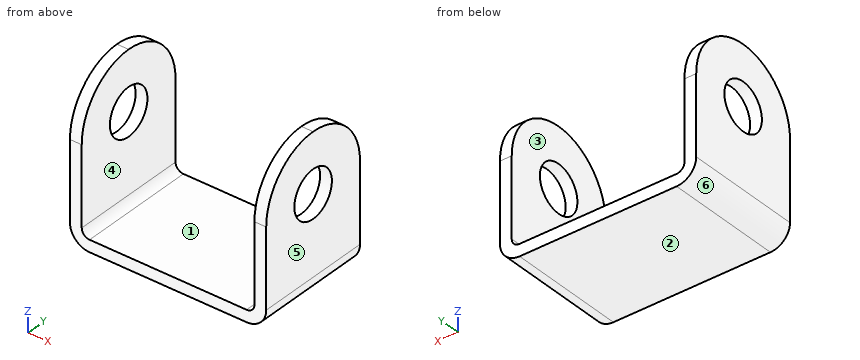
```python
from build123d import *

# Parameters (mm, degrees)
SKICA1_W                      = 50
SKICA1_H                      = 30
P_IDAT_VYSUNUT_M1_DEPTH       = 40
ZAOBLIT1_R                    = 15
ODEBRAT_VYSUNUT_M1_DEPTH      = 50.497474683
ODEBRAT_VYSUNUT_M1_DEPTH_BACK = 50.497474683
SKICA2_W                      = 44
SKICA2_H                      = 50
ZAOBLIT2_R                    = 2
ZAOBLIT3_R                    = 5
SKICA3_R                      = 6
ODEBRAT_VYSUNUT_M2_DEPTH      = 66.76473219


with BuildPart() as part:
    # Skica1 → Přidat vysunutím1 (new body)
    with BuildSketch(Plane.XY):
        Rectangle(SKICA1_W, SKICA1_H)
    extrude(amount=P_IDAT_VYSUNUT_M1_DEPTH)

    # Zaoblit1
    zaoblit1_edges = [part.edges().sort_by_distance(p)[0] for p in [
        (0, -15, 40),
        (0, 15, 40),
    ]]
    fillet(zaoblit1_edges, radius=ZAOBLIT1_R - 0.0001)  # a hair under: the kernel refuses the full size

    # Skica2 → Odebrat vysunutím1 (cut, two sides: drawn at the far end of the back side and taken through both)
    with BuildSketch(Plane(origin=(0, 0, 0), x_dir=(1, 0, 0), z_dir=(0, 1, 0)).offset(-ODEBRAT_VYSUNUT_M1_DEPTH_BACK)):
        with Locations((0, -28)):
            Rectangle(SKICA2_W, SKICA2_H)
    extrude(amount=ODEBRAT_VYSUNUT_M1_DEPTH + ODEBRAT_VYSUNUT_M1_DEPTH_BACK, mode=Mode.SUBTRACT)

    # Zaoblit2
    zaoblit2_edges = [part.edges().sort_by_distance(p)[0] for p in [
        (-22, 0, 3),
        (22, 0, 3),
    ]]
    fillet(zaoblit2_edges, radius=ZAOBLIT2_R)

    # Zaoblit3
    zaoblit3_edges = [part.edges().sort_by_distance(p)[0] for p in [
        (25, 0, 0),
        (-25, 0, 0),
    ]]
    fillet(zaoblit3_edges, radius=ZAOBLIT3_R)

    # Skica3 → Odebrat vysunutím2 (cut, through all)
    with BuildSketch(Plane(origin=(25, 0, 0), x_dir=(0, 0, -1), z_dir=(1, 0, 0))):
        with Locations(Location((-25, 0, 0), (0, 0, 90))):
            Circle(SKICA3_R)
    extrude(amount=-ODEBRAT_VYSUNUT_M2_DEPTH, mode=Mode.SUBTRACT)


solid = part.part
```
The model under review builds one solid part; all positions refer to its coordinate system, in mm. Face numbers are marked on the shaded views. A direction names the side the tool comes from. Give positions to 0.01 mm unless a question says otherwise; leave off trailing zeros. Write each loop counter-clockwise with the first axis right and the second up, starting at its lowest first coordinate (ties: lowest second). Pieces come first, ordered by that corner, then holes.
(1) To check wall thickness, follow L1, parallel to X at y = -2.5, z = 10.5; L2, parallel to X at y = 5, z = 4; L3, parallel to Z at x = 0, y = -12.5. State the ranges of each line that lie inside material, in increasing order.
(2) Consider section D-D, the plane x = -5.5. Give the boundary of the cut face in (y, z), and give its area (3 significant figures).
(3) Tool access review of the marked faces 1 and 2: name each direction out of +Z, -Z, +X, -X, +Y, -Y from which nothing blocks a thin tool from reaching the whole face with its end or side.
(4) Consider section C-C, the plane z = 29.5. Give the boundary of the cut face in (x, y), and give its area (3 significant figures).
(5) For P1, Ø7, axis at y = 0, z = 25, coming from the -X side; P2, Ø9, axis at y = 3.5, z = 24, coming from the +X side, all flat-tipped, find the tip position at first contact; note any pin that passes through.
(6) The part is to be moulded in two halves that separate along X. For the marked faces 3, 4, 5 and 6, say which applies: released by +X, released by -X, zero draft, split by the parting line, or undercut.
(7) Consider section B-B, the plane y = 1.5. Give the boundary of the cut face in (x, z).
(8) Consider section A-A, the plane z = 15. Give the boundary of the cut face in (x, y).
Returned:
1. L1: x = -25 to -22, 22 to 25
1. L2: x = -24.9 to -21.73, 21.73 to 24.9
1. L3: z = 0 to 3
2. outline: (-15, 0) - (15, 0) - (15, 3) - (-15, 3) - close
2. area: 90.0 mm2
3. face 1: +Z, +Y, -Y
3. face 2: -Z, +X, -X, +Y, -Y
4. outline: (-25, -14.31) - (-22, -14.31) - (-22, -3.97) - (-25, -3.97) - close; (-25, 3.97) - (-22, 3.97) - (-22, 14.31) - (-25, 14.31) - close; (22, -14.31) - (25, -14.31) - (25, -3.97) - (22, -3.97) - close; (22, 3.97) - (25, 3.97) - (25, 14.31) - (22, 14.31) - close
4. area: 124 mm2
5. P1: passes through
5. P2: stops at x = 25
6. face 3: undercut
6. face 4: undercut
6. face 5: released by +X
6. face 6: released by -X
7. outline: (-25, 5) arc R5 ccw to (-20, 0) - (20, 0) arc R5 ccw to (25, 5) - (25, 19.19) - (22, 19.19) - (22, 5) arc R2 cw to (20, 3) - (-20, 3) arc R2 cw to (-22, 5) - (-22, 19.19) - (-25, 19.19) - close; (-25, 30.81) - (-22, 30.81) - (-22, 39.92) - (-25, 39.92) - close; (22, 30.81) - (25, 30.81) - (25, 39.92) - (22, 39.92) - close
8. outline: (-25, -15) - (-22, -15) - (-22, 15) - (-25, 15) - close; (22, -15) - (25, -15) - (25, 15) - (22, 15) - close
